The listing builds one solid part. Answer for the finished solid, in the listing's coordinates (mm). A direction names the side the tool comes from. Coordinates: 2 decimals unless noted, no trailing zeros. Loops run counter-clockwise (first coordinate to the right, second up) from the corner with the lowest first, then second, coordinate; pieces in that order, holes last. Notation, with made-up numbers: (75, 36) - (122, 36) arc R15 cw to (122, 59) - close; hole circle Ø9 at (29, 32). An arc over 180 degrees is marked (long way). Put each result on its own line as item: value.
```python
from build123d import *

# Parameters (mm, degrees)
SALIENTE_EXTRUIR2_DEPTH      = 10
SALIENTE_EXTRUIR2_DEPTH_BACK = 2
CROQUIS1_R                   = 4


with BuildPart() as part:
    # Croquis1 → Saliente-Extruir2 (new, two sides: drawn at the far end of the back side and taken through both)
    with BuildSketch(Plane.XY.offset(-SALIENTE_EXTRUIR2_DEPTH_BACK)):
        with BuildLine():
            Line((-94, -100), (94, -100))
            ThreePointArc((94, -100), (98.242640687, -98.242640687), (100, -94))
            Line((100, -94), (100, 94))
            ThreePointArc((100, 94), (98.242640687, 98.242640687), (94, 100))
            Line((94, 100), (-94, 100))
            ThreePointArc((-94, 100), (-98.242640687, 98.242640687), (-100, 94))
            Line((-100, 94), (-100, -94))
            ThreePointArc((-100, -94), (-98.242640687, -98.242640687), (-94, -100))
        make_face()
        with Locations((-85.874076582, 85.874076582)):
            Circle(CROQUIS1_R, mode=Mode.SUBTRACT)
        with Locations((85.874076582, 85.874076582)):
            Circle(CROQUIS1_R, mode=Mode.SUBTRACT)
        with Locations((85.874076582, -85.874076582)):
            Circle(CROQUIS1_R, mode=Mode.SUBTRACT)
        with Locations((-85.874076582, -85.874076582)):
            Circle(CROQUIS1_R, mode=Mode.SUBTRACT)
        with BuildLine():
            Line((-78.475041975, 54.708172492), (-13.195035121, 54.708172492))
            ThreePointArc((-13.195035121, 54.708172492), (-8.952394434, 56.465531805), (-7.195035121, 60.708172492))
            Line((-7.195035121, 60.708172492), (-7.195035121, 68.708172492))
            ThreePointArc((-7.195035121, 68.708172492), (-8.952394434, 72.95081318), (-13.195035121, 74.708172492))
            Line((-13.195035121, 74.708172492), (-78.475041975, 74.708172492))
            ThreePointArc((-78.475041975, 74.708172492), (-82.717682662, 72.95081318), (-84.475041975, 68.708172492))
            Line((-84.475041975, 68.708172492), (-84.475041975, 60.708172492))
            ThreePointArc((-84.475041975, 60.708172492), (-82.717682662, 56.465531805), (-78.475041975, 54.708172492))
        make_face(mode=Mode.SUBTRACT)
        with BuildLine():
            Line((-78.475041975, 11.984829536), (-13.195035121, 11.984829536))
            ThreePointArc((-13.195035121, 11.984829536), (-8.952394434, 13.742188849), (-7.195035121, 17.984829536))
            Line((-7.195035121, 17.984829536), (-7.195035121, 25.984829536))
            ThreePointArc((-7.195035121, 25.984829536), (-8.952394434, 30.227470223), (-13.195035121, 31.984829536))
            Line((-13.195035121, 31.984829536), (-78.475041975, 31.984829536))
            ThreePointArc((-78.475041975, 31.984829536), (-82.717682662, 30.227470223), (-84.475041975, 25.984829536))
            Line((-84.475041975, 25.984829536), (-84.475041975, 17.984829536))
            ThreePointArc((-84.475041975, 17.984829536), (-82.717682662, 13.742188849), (-78.475041975, 11.984829536))
        make_face(mode=Mode.SUBTRACT)
        with BuildLine():
            Line((-78.208559193, -31.718346754), (-12.928552339, -31.718346754))
            ThreePointArc((-12.928552339, -31.718346754), (-8.685911652, -29.960987441), (-6.928552339, -25.718346754))
            Line((-6.928552339, -25.718346754), (-6.928552339, -17.718346754))
            ThreePointArc((-6.928552339, -17.718346754), (-8.685911652, -13.475706067), (-12.928552339, -11.718346754))
            Line((-12.928552339, -11.718346754), (-78.208559193, -11.718346754))
            ThreePointArc((-78.208559193, -11.718346754), (-82.45119988, -13.475706067), (-84.208559193, -17.718346754))
            Line((-84.208559193, -17.718346754), (-84.208559193, -25.718346754))
            ThreePointArc((-84.208559193, -25.718346754), (-82.45119988, -29.960987441), (-78.208559193, -31.718346754))
        make_face(mode=Mode.SUBTRACT)
        with BuildLine():
            Line((-78.475041975, -74.888557479), (-13.195035121, -74.888557479))
            ThreePointArc((-13.195035121, -74.888557479), (-8.952394434, -73.131198166), (-7.195035121, -68.888557479))
            Line((-7.195035121, -68.888557479), (-7.195035121, -60.888557479))
            ThreePointArc((-7.195035121, -60.888557479), (-8.952394434, -56.645916792), (-13.195035121, -54.888557479))
            Line((-13.195035121, -54.888557479), (-78.475041975, -54.888557479))
            ThreePointArc((-78.475041975, -54.888557479), (-82.717682662, -56.645916792), (-84.475041975, -60.888557479))
            Line((-84.475041975, -60.888557479), (-84.475041975, -68.888557479))
            ThreePointArc((-84.475041975, -68.888557479), (-82.717682662, -73.131198166), (-78.475041975, -74.888557479))
        make_face(mode=Mode.SUBTRACT)
        with BuildLine():
            Line((13.461517903, 11.984829536), (78.208559193, 11.984829536))
            ThreePointArc((78.208559193, 11.984829536), (82.45119988, 13.742188849), (84.208559193, 17.984829536))
            Line((84.208559193, 17.984829536), (84.208559193, 25.984829536))
            ThreePointArc((84.208559193, 25.984829536), (82.45119988, 30.227470223), (78.208559193, 31.984829536))
            Line((78.208559193, 31.984829536), (13.461517903, 31.984829536))
            ThreePointArc((13.461517903, 31.984829536), (9.218877216, 30.227470223), (7.461517903, 25.984829536))
            Line((7.461517903, 25.984829536), (7.461517903, 17.984829536))
            ThreePointArc((7.461517903, 17.984829536), (9.218877216, 13.742188849), (13.461517903, 11.984829536))
        make_face(mode=Mode.SUBTRACT)
        with BuildLine():
            Line((13.461517903, 54.708172492), (78.208559193, 54.708172492))
            ThreePointArc((78.208559193, 54.708172492), (82.45119988, 56.465531805), (84.208559193, 60.708172492))
            Line((84.208559193, 60.708172492), (84.208559193, 68.708172492))
            ThreePointArc((84.208559193, 68.708172492), (82.45119988, 72.95081318), (78.208559193, 74.708172492))
            Line((78.208559193, 74.708172492), (13.461517903, 74.708172492))
            ThreePointArc((13.461517903, 74.708172492), (9.218877216, 72.95081318), (7.461517903, 68.708172492))
            Line((7.461517903, 68.708172492), (7.461517903, 60.708172492))
            ThreePointArc((7.461517903, 60.708172492), (9.218877216, 56.465531805), (13.461517903, 54.708172492))
        make_face(mode=Mode.SUBTRACT)
        with BuildLine():
            Line((13.728000685, -31.718346754), (78.475041975, -31.718346754))
            ThreePointArc((78.475041975, -31.718346754), (82.717682662, -29.960987441), (84.475041975, -25.718346754))
            Line((84.475041975, -25.718346754), (84.475041975, -17.718346754))
            ThreePointArc((84.475041975, -17.718346754), (82.717682662, -13.475706067), (78.475041975, -11.718346754))
            Line((78.475041975, -11.718346754), (13.728000685, -11.718346754))
            ThreePointArc((13.728000685, -11.718346754), (9.485359998, -13.475706067), (7.728000685, -17.718346754))
            Line((7.728000685, -17.718346754), (7.728000685, -25.718346754))
            ThreePointArc((7.728000685, -25.718346754), (9.485359998, -29.960987441), (13.728000685, -31.718346754))
        make_face(mode=Mode.SUBTRACT)
        with BuildLine():
            Line((13.461517903, -74.888557479), (78.208559193, -74.888557479))
            ThreePointArc((78.208559193, -74.888557479), (82.45119988, -73.131198166), (84.208559193, -68.888557479))
            Line((84.208559193, -68.888557479), (84.208559193, -60.888557479))
            ThreePointArc((84.208559193, -60.888557479), (82.45119988, -56.645916792), (78.208559193, -54.888557479))
            Line((78.208559193, -54.888557479), (13.461517903, -54.888557479))
            ThreePointArc((13.461517903, -54.888557479), (9.218877216, -56.645916792), (7.461517903, -60.888557479))
            Line((7.461517903, -60.888557479), (7.461517903, -68.888557479))
            ThreePointArc((7.461517903, -68.888557479), (9.218877216, -73.131198166), (13.461517903, -74.888557479))
        make_face(mode=Mode.SUBTRACT)
    extrude(amount=SALIENTE_EXTRUIR2_DEPTH + SALIENTE_EXTRUIR2_DEPTH_BACK)


solid = part.part
```
1) For a pull along Y with two mould halves and no side action, classify faces 1 (the face through (-98.196, 98.289, 3.916)), 2 (the face through (45, 11.985, 4)), 3 (the face through (-1, 1, -2)), 4 (the face through (82.404, 13.696, 3.916)) as pulls with the +Y half, pulls with the -Y half, needs draft (parallel to the pull), parting line crosses it, or undercut.
Found:
face 1: pulls with the +Y half
face 2: undercut
face 3: needs draft
face 4: undercut
2) For faces 5 (the face through (98.196, -98.289, 3.916)), 6 (the face through (9.439, -29.914, 3.916)), determine the directions among +Z, -Z, +X, -X, +Y, -Y from which every point of the face is accessible in a straight line to the end or side of a thin tool.
Found:
face 5: +Z, -Z, +X, -Y
face 6: +Z, -Z
3) The part is cut by section B-B (z = 4). State how many separate pieces and enclosed holes the cut face has, and give its area (3 significant figures).
Found:
separate pieces: 1
enclosed holes: 12
area: 27,700 mm^2
4) The part is cut by section A-A (x = -55.5). Give the vertices of the cut face in (y, z).
Found:
outline: (-100, -2) - (-74.89, -2) - (-74.89, 10) - (-100, 10) - close; (-54.89, -2) - (-31.72, -2) - (-31.72, 10) - (-54.89, 10) - close; (-11.72, -2) - (11.98, -2) - (11.98, 10) - (-11.72, 10) - close; (31.98, -2) - (54.71, -2) - (54.71, 10) - (31.98, 10) - close; (74.71, -2) - (100, -2) - (100, 10) - (74.71, 10) - close
5) Straight lines are drawn through the part: L1, parallel to X at y = -24, z = 8.75; L2, parallel to Y at x = 79, z = 3.75; L3, parallel to Y at x = -25, z = 2.25. For each, find the intervals that lie inside material, in ascending order. Write a range as [from, to].
Found:
L1: x = [-100, -84.21], [-6.93, 7.73], [84.48, 100]
L2: y = [-100, -74.84], [-54.94, -31.7], [-11.74, 12.04], [31.93, 54.76], [74.66, 100]
L3: y = [-100, -74.89], [-54.89, -31.72], [-11.72, 11.98], [31.98, 54.71], [74.71, 100]
6) This flat-tipped pin is pushed along its axis until it touches: pin 1 (10.5 mm diameter, centred on x = -85.87, y = 85.87, fed in from +Z). Where does it stop, or does it pass through?
Found:
pin 1: stops at z = 10
